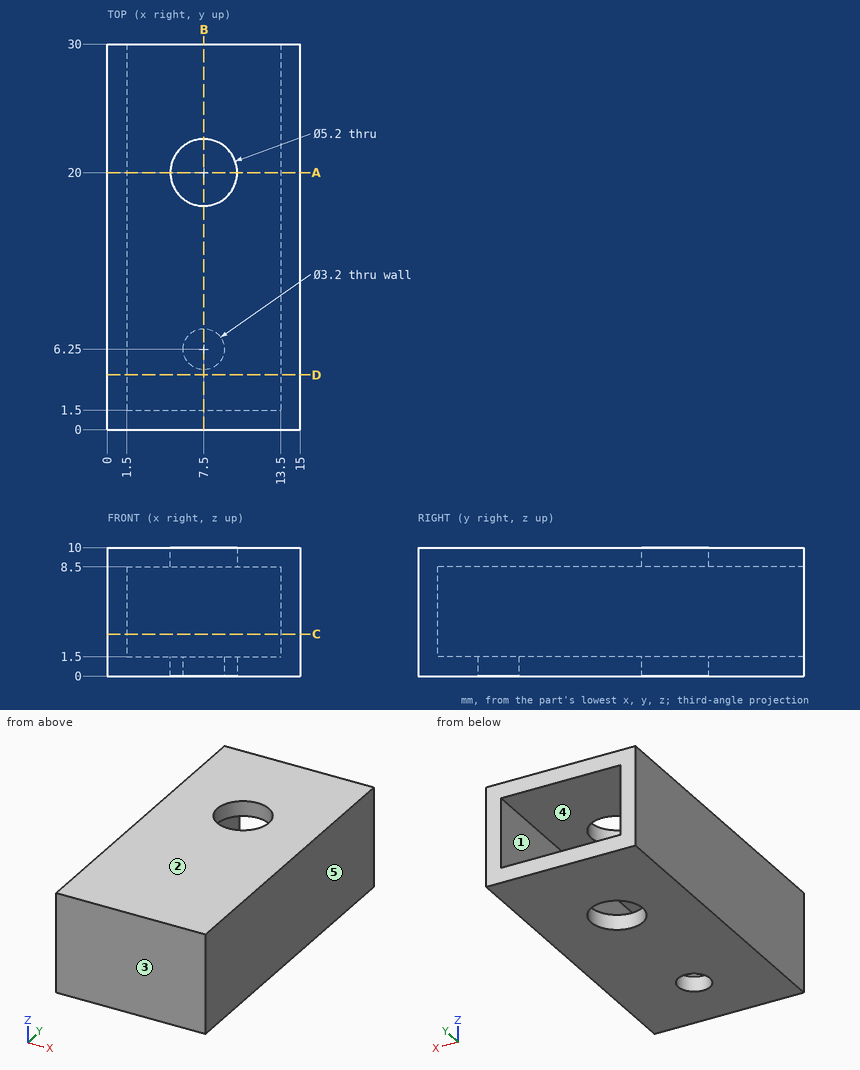
Design review of the part shown in the three views and the two pictorial views. Dimensions are in mm from the part's minimum x, y and z. A direction names the side the tool comes from. Round coordinates to 2 decimals unless told otherwise and drop trailing zeros. Order: outer loops, then holes, each group sorted by start corner. A loop starts at its lowest first (then second) coordinate and runs counter-clockwise, first axis right, second up. Notation, with made-up numbers: (85, 40.5) - (122, 40.5) arc R14 ccw to (122, 44.5) - close; hole circle Ø6 at (-39, 84.5). An arc over 180 degrees is marked (long way). Answer in a Markdown table with one row per item.
(1) For line 1 (Y direction, x = 7.5, z = 1); line 2 (Z direction, x = 10.75, y = 11.75); line 3 (X direction, y = 17, z = 2.75), list the stretches that pass through material, from the lowest coordinate up. Write a range as from..to.
Result set:
| item | result |
|---|---|
| line 1 | y = 0..4.65, 7.85..17.4, 22.6..30 |
| line 2 | z = 0..1.5, 8.5..10 |
| line 3 | x = 0..1.5, 13.5..15 |
(2) Take a section at C-C on z = 3.25. Write out the cut boundary in (x, y), plus the area to 3 significant figures.
Result set:
| item | result |
|---|---|
| outline | (0, 0) - (15, 0) - (15, 30) - (13.5, 30) - (13.5, 1.5) - (1.5, 1.5) - (1.5, 30) - (0, 30) - close |
| area | 108 mm2 |
(3) Mouldability with a two-part tool opening along X and no side actions: class the marked faces 3, 4 and 5 as released by +X, released by -X, zero draft, split by the parting line, or undercut.
Result set:
| item | result |
|---|---|
| face 3 | zero draft |
| face 4 | undercut |
| face 5 | released by +X |
(4) Clearance check with flat-ended pins moving along their axes: P1, Ø3.5, axis at x = 9, z = 5, coming from the +Y side; P2, Ø4, axis at x = 7.5, y = 20, coming from the +Z side; P3, Ø8.5, axis at x = 7.5, y = 20, coming from the -Z side. State where each tip first meets the part, or that it passes through.
Result set:
| item | result |
|---|---|
| P1 | stops at y = 1.5 |
| P2 | passes through |
| P3 | stops at z = 0 |
(5) Take a section at A-A on y = 20. Write out the cut boundary in (x, z).
Result set:
| item | result |
|---|---|
| outline | (0, 0) - (4.9, 0) - (4.9, 1.5) - (1.5, 1.5) - (1.5, 8.5) - (4.9, 8.5) - (4.9, 10) - (0, 10) - close; (10.1, 0) - (15, 0) - (15, 10) - (10.1, 10) - (10.1, 8.5) - (13.5, 8.5) - (13.5, 1.5) - (10.1, 1.5) - close |
(6) Take a section at B-B on x = 7.5. Write out the cut boundary in (y, z).
Result set:
| item | result |
|---|---|
| outline | (0, 0) - (4.65, 0) - (4.65, 1.5) - (1.5, 1.5) - (1.5, 8.5) - (17.4, 8.5) - (17.4, 10) - (0, 10) - close; (7.85, 0) - (17.4, 0) - (17.4, 1.5) - (7.85, 1.5) - close; (22.6, 0) - (30, 0) - (30, 1.5) - (22.6, 1.5) - close; (22.6, 8.5) - (30, 8.5) - (30, 10) - (22.6, 10) - close |
(7) Machinability: for the marked faces 1 and 2, which of the approach directions +Z, -Z, +X, -X, +Y, -Y give a long, thin tool a straight path to every point of the face, cutting with its end or side? Answer none if there is none.
Result set:
| item | result |
|---|---|
| face 1 | +Y |
| face 2 | +Z, +X, -X, +Y, -Y |
(8) Take a section at D-D on y = 4.25. Write out the cut boundary in (x, z).
Result set:
| item | result |
|---|---|
| outline | (0, 0) - (15, 0) - (15, 10) - (0, 10) - close; hole (1.5, 1.5) - (13.5, 1.5) - (13.5, 8.5) - (1.5, 8.5) - close |
